Geometry check sheet. Reference: the model listing, model coordinates, mm. Round coordinates to 2 decimals unless told otherwise and drop trailing zeros. Loops run counter-clockwise (first coordinate to the right, second up) from the corner with the lowest first, then second, coordinate; pieces in that order, holes last. Notation, with made-up numbers: (64, 56) - (89, 56) arc R33 ccw to (89, 91) - close; hole circle Ø10 at (81.25, -16). An arc over 180 degrees is marked (long way). Write item = value, one per line.
```python
from build123d import *

# Parameters (mm, degrees)
BOX001_W               = 10
BOX001_H               = 10
BOX001_DEPTH           = 10
BOX001_PLACEMENT_ANGLE = 1
BOX_W                  = 10
BOX_H                  = 10
BOX_DEPTH              = 10


with BuildPart() as obj1:
    # Box001 → Box001 (new body)
    with BuildSketch(Plane.XY):
        with Locations((5, 5)):
            Rectangle(BOX001_W, BOX001_H)
    extrude(amount=BOX001_DEPTH)


with BuildPart() as obj1_1:
    # Box001 placement: moved
    add(obj1.part.moved(Location((3, 3, 3))).rotate(Axis((3, 3, 3), (0, 0, -1)), BOX001_PLACEMENT_ANGLE))


with BuildPart() as cut:
    # Box → Box (new body)
    with BuildSketch(Plane.XY):
        with Locations((5, 5)):
            Rectangle(BOX_W, BOX_H)
    extrude(amount=BOX_DEPTH)

    # Cut: cut obj1
    add(obj1_1.part, mode=Mode.SUBTRACT)


solid = cut.part
```
(1) Gauge pin test, flat ends, axial feed: pin 1 (2 mm diameter, centred on y = 6.5, z = 4.5, fed in from +X); pin 2 (2 mm diameter, centred on y = 4.5, z = 6, fed in from +X); pin 3 (2 mm diameter, centred on x = 7.5, y = 7, fed in from +Z). Record the tip position at first contact, or that the pin passes through.
Answers follow:
pin_1 = 3.08
pin_2 = 3.04
pin_3 = 3
(2) Scan lines: L1, parallel to Z at x = 6.75, y = 6; L2, parallel to X at y = 9.75, z = 7.75; L3, parallel to Y at x = 9.75, z = 4.75. Record each from-to range of solid material in increasing order. Write a range as [from, to].
Answers follow:
L1 = [0, 3]
L2 = [0, 3.12]
L3 = [0, 2.88]
(3) Section check A-A (z = 8). Enter the section's corners in (x, y).
Answers follow:
outline = (0, 0) - (10, 0) - (10, 2.88) - (3, 3) - (3.12, 10) - (0, 10) - close
(4) Section check B-B (y = 3.75). Enter the section's corners in (x, z).
Answers follow:
outline = (0, 0) - (10, 0) - (10, 3) - (3.01, 3) - (3.01, 10) - (0, 10) - close
